Geometry check sheet. Reference: the model listing, model coordinates, mm. Give positions to 0.01 mm unless a question says otherwise; leave off trailing zeros. Write each loop counter-clockwise with the first axis right and the second up, starting at its lowest first coordinate (ties: lowest second). Pieces come first, ordered by that corner, then holes. Notation, with made-up numbers: (5.25, -22) -> (29.25, -22) arc R8 cw to (29.25, -15) -> close; hole circle Ø8 at (84, 0). An arc over 180 degrees is marked (long way). One line per item, written item: value.
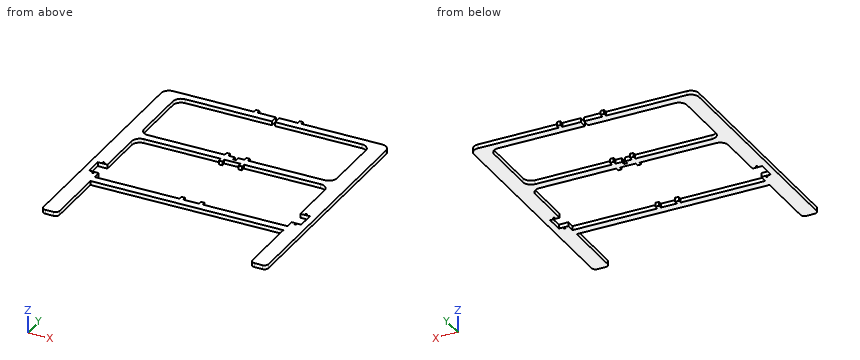
from build123d import *

# Parameters (mm, degrees)
SKETCH1_R           = 1
SKETCH1_W           = 4.5
SKETCH1_H           = 4.5
BOSS_EXTRUDE1_DEPTH = 2.5


with BuildPart() as part:
    # Sketch1 → Boss-Extrude1 (new body, symmetric)
    with BuildSketch(Plane.XY):
        with BuildLine():
            Line((-140, 90), (-140, -195))
            ThreePointArc((-140, -195), (-138.535533906, -198.535533906), (-135, -200))
            Line((-135, -200), (-125, -200))
            ThreePointArc((-125, -200), (-121.464466094, -198.535533906), (-120, -195))
            Line((-120, -195), (-120, -100))
            Line((-120, -100), (-132, -100))
            Line((-132, -100), (-132, -79))
            Line((-132, -79), (-120, -79))
            Line((-120, -79), (-120, -20))
            ThreePointArc((-120, -20), (-117.071067812, -12.928932188), (-110, -10))
            Line((-110, -10), (0, -10))
            Line((0, -10), (0, -5))
            Line((0, -5), (-2, -5))
            Line((-2, -5), (-2, 0))
            Line((-2, 0), (-110, 0))
            ThreePointArc((-110, 0), (-117.071067812, 2.928932188), (-120, 10))
            Line((-120, 10), (-120, 80))
            ThreePointArc((-120, 80), (-117.071067812, 87.071067812), (-110, 90))
            Line((-110, 90), (-2, 90))
            Line((-2, 90), (-2, 100))
            Line((-2, 100), (-120, 100))
            Line((-120, 100), (-130, 100))
            ThreePointArc((-130, 100), (-137.071067812, 97.071067812), (-140, 90))
        make_face()
        with Locations((-126, -77)):
            Circle(SKETCH1_R, mode=Mode.SUBTRACT)
        with Locations((-126, -102)):
            Circle(SKETCH1_R, mode=Mode.SUBTRACT)
        Polygon((-14.5, -110), (-120, -110), (-120, -120), (0, -120), (0, -110), (-10, -110), align=None)
        with Locations((-12.25, -107.75)):
            Rectangle(SKETCH1_W, SKETCH1_H)
        with Locations((-12.25, 2.25)):
            Rectangle(SKETCH1_W, SKETCH1_H)
        with Locations((-12.25, -12.25)):
            Rectangle(SKETCH1_W, SKETCH1_H)
        with Locations((-27.25, 102.25)):
            Rectangle(SKETCH1_W, SKETCH1_H)
    boss_extrude1 = extrude(amount=BOSS_EXTRUDE1_DEPTH, both=True)

    # Mirror1: Boss-Extrude1 across plane
    add(boss_extrude1.mirror(Plane(origin=(0, 0, 0), x_dir=(0, 0, 1), z_dir=(1, 0, 0))))


solid = part.part
1) Sectioned sample at A-A on y = 76. Record the cut outline in (x, z).
Verdict:
outline: (-140, -2.5) -> (-120, -2.5) -> (-120, 2.5) -> (-140, 2.5) -> close; (120, -2.5) -> (140, -2.5) -> (140, 2.5) -> (120, 2.5) -> close
2) Scan lines: probe 1 along Y at (x, z) = (-55, 2.05); probe 2 along X at (y, z) = (-77, -1); probe 3 along Y at (x, z) = (126, 1.3). Record each from-to range of solid material in increasing order.
Verdict:
probe 1: -120 to -110, -10 to 0, 90 to 100
probe 2: -140 to -127, -125 to -120, 120 to 125, 127 to 140
probe 3: -200 to -103, -101 to -100, -79 to -78, -76 to 100
3) Depth check by flat-ended pin: pin 1 Ø1.3 at (x, z) = (-13.5, 1) entering from -Y; pin 2 Ø1.5 at (x, z) = (-16, 0) entering from +Y. Enter the tip coordinate at first touch or a pass-through.
Verdict:
pin 1: y = -120
pin 2: y = 100
4) Sectioned sample at B-B on x = -77.5. Record the cut outline in (y, z).
Verdict:
outline: (-120, -2.5) -> (-110, -2.5) -> (-110, 2.5) -> (-120, 2.5) -> close; (-10, -2.5) -> (0, -2.5) -> (0, 2.5) -> (-10, 2.5) -> close; (90, -2.5) -> (100, -2.5) -> (100, 2.5) -> (90, 2.5) -> close
5) Sectioned sample at C-C on z = -0.8. Give the number of separate pieces and of enclosed holes in the cut face, plus the area to 3 significant figures.
Verdict:
separate pieces: 1
enclosed holes: 5
area: 18,800 mm^2
